Geometry check sheet. Reference: the model listing, model coordinates, mm. A direction names the side the tool comes from. Give positions to 0.01 mm unless a question says otherwise; leave off trailing zeros. Loops run counter-clockwise (first coordinate to the right, second up) from the corner with the lowest first, then second, coordinate; pieces in that order, holes last. Notation, with made-up numbers: (29.25, 15.5) -> (86.25, 15.5) arc R19 ccw to (86.25, 45.5) -> close; hole circle Ø9 at (-28, -36). An arc over 180 degrees is marked (long way). One line per item, written item: value. Start each with the question number.
(1) Sectioned sample at B-B, the plane z = -43. Record the cut outline in (x, y), then the cut area to 3 significant figures.
(2) Draft check along X on faces 4 (the face through (-43, 0, -38)), 5 (the face through (-185.29, -13.25, -97.27)), 6 (the face through (-116.5, -13.3, -60.8)). Enter one of: pulls with the +X half, pulls with the -X half, needs draft (parallel to the pull), parting line crosses it, or undercut.
(3) Sectioned sample at A-A, the plane x = -182. Record the cut outline in (y, z).
(4) Tool access check on faces 1 (the face through (-30.48, -12, -29)), 2 (the face through (-13, -9, -55.88)), 3 (the face through (-79, -17, -30.353)). Record the directions out of +Z, -Z, +X, -X, +Y, -Y that give a thin tool (end or side, any length) a straight path to the whole face; none if there is none.
(5) Gauge pin test, flat ends, axial feed: pin 1 Ø4 at (y, z) = (-14.5, -21.5) entering from -X; pin 2 Ø1 at (x, y) = (-80, -17.5) entering from +Z; pin 3 Ø3 at (y, z) = (-5, -86) entering from -X; pin 4 Ø8 at (x, y) = (-86, -7.5) entering from -Z. Record the tip position at first contact, or that the pin passes through.
(6) Sectioned sample at D-D, the plane x = -15. Record the cut outline in (y, z).
(7) Scan lines: line 1 along X through (y, z) = (-15, -24); line 2 along Z through (x, y) = (-155, -17); line 3 along Z through (x, y) = (-166, -13.5). Record each from-to range of solid material in increasing order. Write a range as from..to.
(8) Sectioned sample at C-C, the plane x = -63.5. Record the cut outline in (y, z) (1 decimal), then the cut area to 3 significant figures.
from build123d import *

# Parameters (mm, degrees)
F1_DEPTH  = 19.05
F3_DEPTH  = 13.97
F5_DEPTH  = 7.62
F7_DEPTH  = 11.43
F8_R      = 7.9375
F9_R      = 1.5875
F10_DEPTH = 4.7625
F11_DEPTH = 19.0510001


# Not quite as in the source:
# - a feature names something its author has since deleted; it is built from what else it names


with BuildPart() as f1:
    # F0 (on Front) → F1 (new body)
    with BuildSketch(Plane.XZ):
        Polygon((0, -55.88), (0, 0), (-30.48, 0), (-30.48, -57.344024155), (-25.4, -55.88), align=None)
        with BuildLine():
            Line((-50.8, -63.2001207751), (-50.8, 0))
            ThreePointArc((-50.8, 0), (-53.8879738976, -1.0462898954), (-55.7039336667, -3.7541664537))
            ThreePointArc((-55.7039336667, -3.7541664537), (-65.0479350522, -20.0515789601), (-81.1885565746, -29.6638811382))
            Line((-81.1885565746, -29.6638811382), (-195.2974379776, -62.5493454446))
            Line((-195.2974379776, -62.5493454446), (-192.8355918237, -71.0916761286))
            Line((-192.8355918237, -71.0916761286), (-119.6156145323, -49.990137667))
            Line((-119.6156145323, -49.990137667), (-113.2851529938, -71.9561308545))
            Line((-113.2851529938, -71.9561308545), (-186.5051302853, -93.057669316))
            Line((-186.5051302853, -93.057669316), (-184.0432841314, -101.6))
            Line((-184.0432841314, -101.6), (-50.8, -63.2001207751))
        make_face()
        Polygon((-30.48, -57.344024155), (-30.48, 0), (-50.8, 0), (-50.8, -63.2001207751), align=None)
    extrude(amount=F1_DEPTH)

    # F2 (on face) → F3 (cut)
    with BuildSketch(Plane.XZ.offset(19.05)):
        Polygon((-30.48, 0), (-50.8, 0), (-50.8, -63.2001207751), (-30.48, -57.344024155), align=None)
    extrude(amount=-F3_DEPTH, mode=Mode.SUBTRACT)

    # F4 (on face) → F5 (cut)
    with BuildSketch(Plane.XZ):
        Polygon((-109.8741311376, -37.9308839061), (-195.2974379776, -62.5493454446), (-184.0432841314, -101.6), (-98.6199772914, -76.9815384615), align=None)
    extrude(amount=F5_DEPTH, mode=Mode.SUBTRACT)

    # F6 (on face) → F7 (cut)
    with BuildSketch(Plane.XZ.offset(19.05)):
        with BuildLine():
            Line((-83.9840349336, -30.353), (-50.8, -30.353))
            Line((-50.8, -30.353), (-50.8, 0))
            ThreePointArc((-50.8, 0), (-53.8879738976, -1.0462898954), (-55.7039336667, -3.7541664537))
            ThreePointArc((-55.7039336667, -3.7541664537), (-66.0773822208, -21.0582659153), (-83.9840349336, -30.353))
        make_face()
    extrude(amount=-F7_DEPTH, mode=Mode.SUBTRACT)

    # F8
    f8_edges = [f1.edges().sort_by_distance(p)[0] for p in [
        (-67.189861, -7.62, -30.353),
    ]]
    fillet(f8_edges, radius=F8_R)

    # F9 (on face) → F10 (cut)
    with BuildSketch(Plane.XZ.offset(19.05)):
        with BuildLine():
            Line((-78.4844835363, -71.1786153846), (-73.6695687, -69.790987112))
            ThreePointArc((-73.6695687, -69.7909871121), (-78.2220260856, -57.0610953752), (-78.0424581585, -43.5428570566))
            ThreePointArc((-78.0424581585, -43.5428570566), (-76.567170767, -38.1173977165), (-74.3094881962, -32.9681306475))
            Line((-74.3094881962, -32.9681306475), (-74.93, -33.1469582596))
            Line((-74.93, -33.1469582596), (-84.154369829, -35.8053638195))
            Line((-84.154369829, -35.8053638195), (-117.3289133872, -45.3660593118))
            Line((-117.3289133872, -45.3660593118), (-107.4815287718, -79.5353820478))
            Line((-107.4815287718, -79.5353820478), (-94.3488119494, -75.7506153846))
            Line((-94.3488119494, -75.7506153846), (-96.9865042571, -66.5981182232))
            Line((-96.9865042571, -66.5981182232), (-81.122175844, -62.0261182232))
            Line((-81.122175844, -62.0261182232), (-78.4844835363, -71.1786153846))
        make_face()
        Polygon((-86.4166477429, -73.4646153846), (-78.4844835363, -71.1786153846), (-81.122175844, -62.0261182232), (-96.9865042571, -66.5981182232), (-94.3488119494, -75.7506153846), align=None)
        with Locations((-93.0564411007, -68.7697198411)):
            Circle(F9_R, mode=Mode.SUBTRACT)
        with Locations((-83.2937774619, -65.9561813796)):
            Circle(F9_R, mode=Mode.SUBTRACT)
        with Locations((-83.2937774619, -65.9561813796)):
            Circle(F9_R)
        with Locations((-93.0564411007, -68.7697198411)):
            Circle(F9_R)
        with BuildLine():
            ThreePointArc((-78.0424581585, -43.5428570566), (-78.2220260856, -57.0610953752), (-73.6695687, -69.7909871121))
            Line((-73.6695687, -69.790987112), (-50.8, -63.2001207751))
            Line((-50.8, -63.2001207751), (-50.8, -53.6799892795))
            Line((-50.8, -53.6799892795), (-74.2742938603, -49.1253072525))
            ThreePointArc((-74.2742938603, -49.1253072525), (-77.3145392982, -47.1144945318), (-78.0424581585, -43.5428570566))
        make_face()
        with BuildLine():
            ThreePointArc((-74.3094881962, -32.9681306475), (-76.567170767, -38.1173977165), (-78.0424581585, -43.5428570566))
            ThreePointArc((-78.0424581585, -43.5428570566), (-72.9114890511, -39.7093483015), (-68.6046509033, -44.45))
            ThreePointArc((-68.6046509033, -44.45), (-70.3372055311, -48.1243485533), (-74.2742938603, -49.1253072525))
            Line((-74.2742938603, -49.1253072525), (-50.8, -53.6799892795))
            Line((-50.8, -53.6799892795), (-50.8, -42.2880161767))
            ThreePointArc((-50.8, -42.2880161767), (-54.8534085622, -36.9235653105), (-56.279986835, -30.353))
            Line((-56.279986835, -30.353), (-65.2352774711, -30.353))
            Line((-65.2352774711, -30.353), (-74.3094881962, -32.9681306475))
        make_face()
        with BuildLine():
            ThreePointArc((-68.6046509033, -44.45), (-72.9114890511, -39.7093483015), (-78.0424581585, -43.5428570566))
            ThreePointArc((-78.0424581585, -43.5428570566), (-77.3145392982, -47.1144945318), (-74.2742938603, -49.1253072525))
            ThreePointArc((-74.2742938603, -49.1253072525), (-70.3372055311, -48.1243485533), (-68.6046509033, -44.45))
        make_face()
        with BuildLine():
            Line((-50.8, -30.353), (-56.279986835, -30.353))
            ThreePointArc((-56.279986835, -30.353), (-54.8534085622, -36.9235653105), (-50.8, -42.2880161767))
            Line((-50.8, -42.2880161767), (-50.8, -30.353))
        make_face()
        with BuildLine():
            Line((-50.8, -28.4059811383), (-56.1527436573, -28.4059811383))
            ThreePointArc((-56.1527436573, -28.4059811383), (-56.2467573472, -29.3775043596), (-56.279986835, -30.353))
            Line((-56.279986835, -30.353), (-50.8, -30.353))
            Line((-50.8, -30.353), (-50.8, -28.4059811383))
        make_face()
        with BuildLine():
            Line((-56.1527436573, -28.4059811383), (-71.4639828579, -28.4059811383))
            ThreePointArc((-71.4639828579, -28.4059811383), (-72.1413197609, -29.3692544852), (-72.7885643692, -30.353))
            Line((-72.7885643692, -30.353), (-65.2352774711, -30.353))
            Line((-65.2352774711, -30.353), (-56.279986835, -30.353))
            ThreePointArc((-56.279986835, -30.353), (-56.2467573472, -29.3775043596), (-56.1527436573, -28.4059811383))
        make_face()
        with BuildLine():
            ThreePointArc((-72.7885643692, -30.353), (-72.1413197609, -29.3692544852), (-71.4639828579, -28.4059811383))
            Line((-71.4639828579, -28.4059811383), (-74.93, -28.4059811383))
            Line((-74.93, -28.4059811383), (-74.93, -30.353))
            Line((-74.93, -30.353), (-72.7885643692, -30.353))
        make_face()
        with BuildLine():
            ThreePointArc((-72.7885643692, -30.353), (-73.5749926059, -31.6454636692), (-74.3094881962, -32.9681306475))
            Line((-74.3094881962, -32.9681306475), (-65.2352774711, -30.353))
            Line((-65.2352774711, -30.353), (-72.7885643692, -30.353))
        make_face()
        with BuildLine():
            Line((-74.93, -33.1469582596), (-74.3094881962, -32.9681306475))
            ThreePointArc((-74.3094881962, -32.9681306475), (-73.5749926059, -31.6454636692), (-72.7885643692, -30.353))
            Line((-72.7885643692, -30.353), (-74.93, -30.353))
            Line((-74.93, -30.353), (-74.93, -33.1469582596))
        make_face()
    extrude(amount=-F10_DEPTH, mode=Mode.SUBTRACT)

    # F9 (on face) → F11 (cut, through all)
    with BuildSketch(Plane.XZ.offset(19.05)):
        with Locations((-83.2937774619, -65.9561813796)):
            Circle(F9_R)
    extrude(amount=-F11_DEPTH, mode=Mode.SUBTRACT)


solid = f1.part
Calculated:
1. outline: (-127.46, -19.05) -> (-109.12, -19.05) -> (-109.12, -14.29) -> (-50.8, -14.29) -> (-50.8, -5.08) -> (-30.48, -5.08) -> (-30.48, -19.05) -> (0, -19.05) -> (0, 0) -> (-108.41, 0) -> (-108.41, -7.62) -> (-127.46, -7.62) -> close
1. area: 1,720 mm2
2. face 4: needs draft
2. face 5: pulls with the -X half
2. face 6: undercut
3. outline: (-19.05, -101.01) -> (-7.62, -101.01) -> (-7.62, -91.76) -> (-19.05, -91.76) -> close; (-19.05, -67.97) -> (-7.62, -67.97) -> (-7.62, -58.72) -> (-19.05, -58.72) -> close
4. face 1: +Z, -Z, -Y
4. face 2: -Z, +X, +Y, -Y
4. face 3: +Z, -X, -Y
5. pin 1: stops at x = -30.48
5. pin 2: stops at z = -30.35
5. pin 3: passes through
5. pin 4: stops at z = -74.5
6. outline: (-19.05, -55.88) -> (0, -55.88) -> (0, 0) -> (-19.05, 0) -> close
7. line 1: x = -30.48..0
7. line 2: z = -93.23..-83.98, -60.19..-50.94
7. line 3: z = -96.4..-87.15, -63.36..-54.11
8. outline: (-14.3, -66.9) -> (0, -66.9) -> (0, -18.4) -> (-7.6, -18.4) -> (-7.6, -22.4) arc R7.9 cw to (-14.3, -30.3) -> close
8. area: 626 mm2
